Input: part model. Units: mm. Frame: model coordinates. A direction names the side the tool comes from. Give positions to 0.01 mm unless a question says otherwise; leave off trailing zeros. Loops run counter-clockwise (first coordinate to the right, second up) from the corner with the lowest first, then second, coordinate; pieces in that order, holes last. Notation, with made-up numbers: M 74.25,-8 L 80.25,-8 A19 ccw 80.25,3 Z; hole C 89,48 d5. An arc over 180 degrees is marked long. One line per item, written item: value. Start each with the question number.
(1) Section C-C on x = -14.5. Output: boundary loops of the cut face in (y, z), plus the area to 3 significant figures.
(2) Ray query, line 1 along Y through (x, z) = (34, 429); line 2 along Z through (x, y) = (54, -818). Return the intervals inside material, ascending. Write a range as from..to.
(3) Pin query (flat end, axial travel): P1, Ø8, axis at x = 9, z = 200, coming from the -Y side; P2, Ø2, axis at x = 19, y = -383, coming from the +Z side; P3, Ø24, axis at y = 21, z = 275, coming from the +X side. Return the tip coordinate at first contact, or that it passes through.
(4) Section A-A on z = 290.5. Output: boundary loops of the cut face in (x, y), plus the area to 3 significant figures.
(5) Pull-direction query (Y, two-part tool) for faces 5 (the flat face through (20.04, -39.39, 49.74)), 6 (the flat face through (20, 20, 5)), 7 (the flat face through (70, -353, -13)), 8 (the flat face through (19.465, 72.273, 47.991)); classes: released by +Y, released by -Y, zero draft, split by the parting line, or undercut.
(6) Section B-B on y = -155. Output: boundary loops of the cut face in (x, z).
(7) Access query for faces 1 (the flat face through (0, 20, 348)), 2 (the flat face through (17.5, -23, 32)), 3 (the flat face through (20, -353, 0)), 4 (the flat face through (5, 20, 348)). Directions: +Z, -Z, +X, -X, +Y, -Y. A direction counts if a zero-diameter tool reaches every point of the face in a straight line with its end or side. Return the directions, or none.
```python
from build123d import *

# Parameters (mm, degrees)
F0_W      = 30
F0_H      = 30
F1_DEPTH  = 700
F2_W      = 100
F2_H      = 1000
F3_DEPTH  = 5
F4_W      = 4.7787350416
F4_H      = 30.3992684931
F4_W_2    = 5.5340740085
F5_DEPTH  = 1000
F7_DEPTH  = 50
F9_DEPTH  = 25
F10_W     = 5
F10_H     = 70
F11_DEPTH = 60
F13_DEPTH = 25


with BuildPart() as f1:
    # F0 (on Top) → F1 (new body)
    with BuildSketch(Plane.XY):
        with BuildLine():
            ThreePointArc((0, 5), (1.4644660941, 1.4644660941), (5, 0))
            Line((5, 0), (35, 0))
            ThreePointArc((35, 0), (38.5355339059, 1.4644660941), (40, 5))
            Line((40, 5), (40, 35))
            ThreePointArc((40, 35), (38.5355339059, 38.5355339059), (35, 40))
            Line((35, 40), (5, 40))
            ThreePointArc((5, 40), (1.4644660941, 38.5355339059), (0, 35))
            Line((0, 35), (0, 5))
        make_face()
        with Locations((20, 20)):
            Rectangle(F0_W, F0_H, mode=Mode.SUBTRACT)
    extrude(amount=F1_DEPTH)

    # F2 (on Top) → F3 (join)
    with BuildSketch(Plane.XY):
        with Locations((20, -360)):
            Rectangle(F2_W, F2_H)
    extrude(amount=F3_DEPTH)

    # F4 (on face) → F5 (join)
    with BuildSketch(Plane(origin=(0, 140, 0), x_dir=(-1, 0, 0), z_dir=(0, 1, 0))):
        with Locations((-67.6106324792, -15.1996342465)):
            Rectangle(F4_W, F4_H)
        with Locations((27.2329629958, -15.1996342465)):
            Rectangle(F4_W_2, F4_H)
    extrude(amount=-F5_DEPTH)

    # F6 (on face) → F7 (join)
    with BuildSketch(Plane(origin=(0, 40, 0), x_dir=(-1, 0, 0), z_dir=(0, 1, 0))):
        Polygon((-17, 5), (-17, 75), (-22, 75), (-22, 5), (-20, 5), align=None)
    extrude(amount=F7_DEPTH)

    # F8 (on face) → F9 (cut)
    with BuildSketch(Plane(origin=(17, 0, 0), x_dir=(0, -1, 0), z_dir=(-1, 0, 0))):
        Polygon((-90, 21.7283517122), (-54.0427826345, 75), (-54.0427826345, 81.2046378851), (-94.0335020423, 81.2046378851), (-94.0335020423, 21.7283517122), align=None)
    extrude(amount=-F9_DEPTH, mode=Mode.SUBTRACT)

    # F10 (on face) → F11 (join)
    with BuildSketch(Plane.XZ):
        with Locations((20, 40)):
            Rectangle(F10_W, F10_H)
    extrude(amount=F11_DEPTH)

    # F12 (on face) → F13 (cut)
    with BuildSketch(Plane.YZ.offset(22.5)):
        Polygon((-60, 25.1793347407), (-18.1954981559, 75), (-60, 75), align=None)
    extrude(amount=-F13_DEPTH, mode=Mode.SUBTRACT)


solid = f1.part
```
Output values:
1. outline: M -860,0 L 140,0 L 140,5 L -860,5 Z
1. area: 5,000 mm²
2. line 1: y = 0..5, 35..40
2. line 2: z = 0..5
3. P1: stops at y = 0
3. P2: stops at z = 5
3. P3: stops at x = 40
4. outline: M 0,5 A5 ccw 5,0 L 35,0 A5 ccw 40,5 L 40,35 A5 ccw 35,40 L 5,40 A5 ccw 0,35 Z; hole M 5,5 L 35,5 L 35,35 L 5,35 Z
4. area: 679 mm²
5. face 5: released by -Y
5. face 6: undercut
5. face 7: zero draft
5. face 8: released by +Y
6. outline: M -30,-30.4 L -24.47,-30.4 L -24.47,0 L 65.22,0 L 65.22,-30.4 L 70,-30.4 L 70,5 L -30,5 Z
7. face 1: +Z, -X, +Y, -Y
7. face 2: +Z, -X, -Y
7. face 3: -Z, +Y, -Y
7. face 4: +Z
